from build123d import *

# Parameters (mm, degrees)
SKETCH1_W           = 3.175
SKETCH1_H           = 3.175
BOSS_EXTRUDE1_DEPTH = 3.175


with BuildPart() as part:
    # Sketch1 → Boss-Extrude1 (new body)
    with BuildSketch(Plane.XY):
        with BuildLine():
            Line((0, 0), (12.7, 0))
            Line((12.7, 0), (12.7, 4.699))
            ThreePointArc((12.7, 4.699), (11.77006403, 6.94406403), (9.525, 7.874))
            Line((9.525, 7.874), (3.175, 7.874))
            ThreePointArc((3.175, 7.874), (0.92993597, 6.94406403), (0, 4.699))
            Line((0, 4.699), (0, 0))
        make_face()
        with Locations((6.35, 4.699)):
            Rectangle(SKETCH1_W, SKETCH1_H, mode=Mode.SUBTRACT)
    extrude(amount=BOSS_EXTRUDE1_DEPTH)


solid = part.part
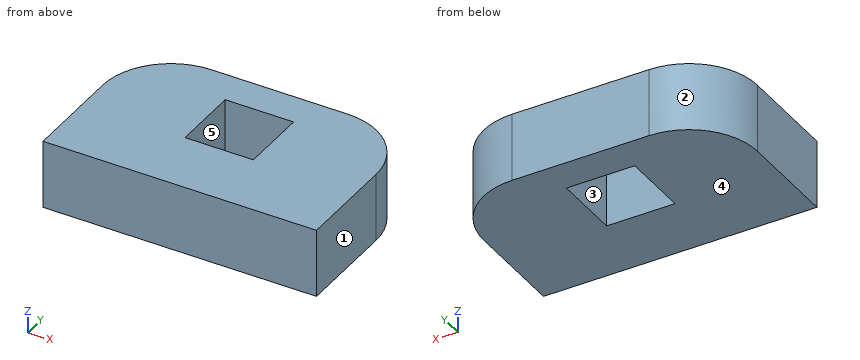
For this review, take the finished solid that the model builds, in its own axes (mm). Face numbers are marked on the shaded views. A direction names the side the tool comes from. Round coordinates to 2 decimals unless told otherwise and drop trailing zeros. Write each loop counter-clockwise with the first axis right and the second up, starting at its lowest first coordinate (ties: lowest second). Pieces come first, ordered by that corner, then holes. Notation, with made-up numbers: (-25.5, -18.5) - (-5.5, -18.5) arc R14 ccw to (-5.5, -0.5) - close; hole circle Ø8 at (32.5, -24.75). An arc over 180 degrees is marked (long way). Use a Markdown table: item, result.
Q1. Clearance check with a flat-ended pin moving along its axis: pin 1 (1 mm diameter, centred on x = 8, z = 2, fed in from -Y). State where the tip first meets the part, or that it passes through.
Derived:
| item | result |
|---|---|
| pin 1 | stops at y = 0 |
Q2. Machinability: for the marked faces 4 and 5, which of the approach directions +Z, -Z, +X, -X, +Y, -Y give a long, thin tool a straight path to every point of the face, cutting with its end or side? Answer none if there is none.
Derived:
| item | result |
|---|---|
| face 4 | -Z, +X, -X, +Y, -Y |
| face 5 | +Z, -Z |
Q3. We need section B-B (y = 3.75). Give the boundary of the cut face in (x, z) (1 decimal), plus the area to 3 significant figures.
Derived:
| item | result |
|---|---|
| outline | (0, 0) - (4.8, 0) - (4.8, 3.2) - (0, 3.2) - close; (7.9, 0) - (12.7, 0) - (12.7, 3.2) - (7.9, 3.2) - close |
| area | 30.2 mm2 |
Q4. The part is to be moulded in two halves that separate along X. For the marked faces 1, 2 and 3, say which applies: pulls with the +X half, pulls with the -X half, needs draft (parallel to the pull), parting line crosses it, or undercut.
Derived:
| item | result |
|---|---|
| face 1 | pulls with the +X half |
| face 2 | pulls with the -X half |
| face 3 | undercut |
Q5. We need section A-A (x = 5.25). Give the boundary of the cut face in (y, z) (1 decimal).
Derived:
| item | result |
|---|---|
| outline | (0, 0) - (3.1, 0) - (3.1, 3.2) - (0, 3.2) - close; (6.3, 0) - (7.9, 0) - (7.9, 3.2) - (6.3, 3.2) - close |
Q6. Wall thickness on line 1 along X through (y, z) = (3.75, 0.6); line 2 along Y through (x, z) = (7.75, 0.3); line 3 along X through (y, z) = (6.25, 2.05): over which ranges is each line inside the solid? List them lowest first.
Derived:
| item | result |
|---|---|
| line 1 | x = 0 to 4.76, 7.94 to 12.7 |
| line 2 | y = 0 to 3.11, 6.29 to 7.87 |
| line 3 | x = 0.4 to 4.76, 7.94 to 12.3 |
Q7. We need section D-D (y = 7.25). Give the boundary of the cut face in (x, z) (3 decimals), plus the area to 3 significant figures.
Derived:
| item | result |
|---|---|
| outline | (1.285, 0) - (11.415, 0) - (11.415, 3.175) - (1.285, 3.175) - close |
| area | 32.2 mm2 |
